from build123d import *

# Parameters (mm, degrees)
F2_W          = 15
F2_H          = 4
F3_DEPTH      = 15.001
F3_DEPTH_BACK = 15.001
F5_DEPTH      = 117.5841784417
F6_R          = 6
F7_DEPTH      = 20.001
F8_R          = 2.5
F9_DEPTH      = 18.501


with BuildPart() as f1:
    # F0 (on Front) → F1 (revolve)
    with BuildSketch(Plane.XZ):
        with BuildLine():
            ThreePointArc((8.2915619759, 12.5), (-7.0931858273, 13.2169101843), (-15, 0))
            Line((-15, 0), (102.5831784417, 0))
            Line((102.5831784417, 0), (102.5831784417, 7.5))
            Line((102.5831784417, 7.5), (72.5831784417, 7.5))
            Line((72.5831784417, 7.5), (55.2915619759, 12.5))
            Line((55.2915619759, 12.5), (8.2915619759, 12.5))
        make_face()
    revolve(axis=Axis((64.8176119516, 0, 0), (1, 0, 0)))

    # F2 (on Front) → F3 (cut, two sides)
    with BuildSketch(Plane.XZ) as f3_sk:
        with Locations((95.0831784417, 5.5)):
            Rectangle(F2_W, F2_H)
        with Locations((95.0831784417, -5.5)):
            Rectangle(F2_W, F2_H)
    extrude(amount=-F3_DEPTH, mode=Mode.SUBTRACT)
    extrude(f3_sk.sketch, amount=F3_DEPTH_BACK, mode=Mode.SUBTRACT)

    # F4 (on face) → F5 (cut, through all)
    with BuildSketch(Plane.YZ.offset(102.5831784417)):
        with BuildLine():
            Line((-10, -11.1803398875), (-10, 11.1803398875))
            ThreePointArc((-10, 11.1803398875), (-15, 0), (-10, -11.1803398875))
        make_face()
        with BuildLine():
            ThreePointArc((10, -11.1803398875), (15, 0), (10, 11.1803398875))
            Line((10, 11.1803398875), (10, -11.1803398875))
        make_face()
    extrude(amount=-F5_DEPTH, mode=Mode.SUBTRACT)

    # F6 (on face) → F7 (cut, through all)
    with BuildSketch(Plane.XZ.offset(10)):
        Circle(F6_R)
    extrude(amount=-F7_DEPTH, mode=Mode.SUBTRACT)

    # F8 (on face) → F9 (cut, through all)
    with BuildSketch(Plane.XY.offset(3.5)):
        with Locations((95.0831784417, 0)):
            Circle(F8_R)
    extrude(amount=-F9_DEPTH, mode=Mode.SUBTRACT)


solid = f1.part
Work out the finished part from the listing and answer in its coordinate system (mm). A direction names the side the tool comes from. Coordinates: 2 decimals unless noted, no trailing zeros. Write each loop counter-clockwise with the first axis right and the second up, starting at its lowest first coordinate (ties: lowest second). Pieces come first, ordered by that corner, then holes.
1. Consider line 1 along Z through (x, y) = (0, 0.5); line 2 along Z through (x, y) = (92.5, 1.25); line 3 along Z through (x, y) = (0, -3). Determine where each line is inside the solid, lowest interval first.
Results list:
line 1: z = -14.99 to -6, 6 to 14.99
line 2: z = -3.5 to 3.5
line 3: z = -14.7 to -6, 6 to 14.7
2. The part is cut by section C-C, the plane x = 53. Write down the section's boundary in (y, z), and give its area (3 significant figures).
Results list:
outline: (-10, -7.5) arc R12.5 ccw to (10, -7.5) - (10, 7.5) arc R12.5 ccw to (-10, 7.5) - close
area: 440 mm2
3. Flat-ended cylindrical pins translate along their axes: pin 1 (6.5 mm diameter, centred on x = 95.08, y = 0, fed in from +Z); pin 2 (2 mm diameter, centred on y = 0.5, z = 5.5, fed in from +X); pin 3 (8 mm diameter, centred on x = 65, y = -5, fed in from -Z); pin 4 (11 mm diameter, centred on x = 0, z = 0, fed in from +Y). Find the tip coordinate at first contact, or state that the pin passes through.
Results list:
pin 1: stops at z = 3.5
pin 2: stops at x = 87.58
pin 3: stops at z = -10.3
pin 4: passes through
4. The part is cut by section A-A, the plane y = 0. Write down the section's boundary in (x, z), and give its area (3 significant figures).
Results list:
outline: (8.29, -12.5) - (55.29, -12.5) - (72.58, -7.5) - (87.58, -7.5) - (87.58, -3.5) - (92.58, -3.5) - (92.58, 3.5) - (87.58, 3.5) - (87.58, 7.5) - (72.58, 7.5) - (55.29, 12.5) - (8.29, 12.5) arc R15 ccw (long way) to start; (97.58, -3.5) - (102.58, -3.5) - (102.58, 3.5) - (97.58, 3.5) - close; hole circle Ø12 at (0, 0)
area: 2,290 mm2
5. For faces 5 (the cylindrical face through (84.04, 6.654, 3.461)), 6 (the flat face through (87.583, 0, 5)), 7 (the cylindrical face through (31.5, -0.2, -12.5)), 8 (the flat face through (87.583, 0, -5)), 9 (the cylindrical face through (92.586, 0.11, 0.049)), determine the directions among +Z, -Z, +X, -X, +Y, -Y from which every point of the face is accessible in a straight line to the end or side of a thin tool.
Results list:
face 5: +X
face 6: +Z, +X, +Y, -Y
face 7: -Z, +X
face 8: -Z, +X, +Y, -Y
face 9: +Z, -Z
6. For a pull along Z with two mould halves and no side action, classify faces 1 (the flat face through (27, 10, 0)), 2 (the conical face through (67.659, -8.848, -1.162)), 3 (the cylindrical face through (-6, 0, 0)), 4 (the cylindrical face through (31.5, 0.2, 12.5)) as +Z half, -Z half, draft (parallel to the pull), parting line (faces both ways), or undercut.
Results list:
face 1: draft
face 2: parting line
face 3: undercut
face 4: +Z half
7. The part is cut by section B-B, the plane z = 0. Write down the section's boundary in (x, y), and give its area (3 significant figures).
Results list:
outline: (-11.18, -10) - (-6, -10) - (-6, 10) - (-11.18, 10) arc R15 ccw to start; (6, -10) - (63.94, -10) - (72.58, -7.5) - (102.58, -7.5) - (102.58, 7.5) - (72.58, 7.5) - (63.94, 10) - (6, 10) - close; hole circle Ø5 at (95.08, 0)
area: 1,900 mm2
